Work out the finished part from the listing and answer in its coordinate system (mm). Face numbers are marked on the shaded views. A direction names the side the tool comes from. Round coordinates to 2 decimals unless told otherwise and drop trailing zeros. Loops run counter-clockwise (first coordinate to the right, second up) from the corner with the lowest first, then second, coordinate; pieces in that order, holes last. Notation, with made-up numbers: (-3, 65.5) - (6, 65.5) arc R7 ccw to (6, 75.5) - close; hole circle Ø11 at (-4.5, -13). An arc over 180 degrees is marked (long way). Answer as CSV lines item,"result". Start each with the question number.
```python
from build123d import *

# Parameters (mm, degrees)
F1_DEPTH = 1500
F2_R     = 120
F3_DEPTH = 715
F4_R     = 50


with BuildPart() as f1:
    # F0 (on Right) → F1 (new body)
    with BuildSketch(Plane.YZ):
        Polygon((250, 724.072175), (0, 724.072175), (-250, 724.072175), (-250, 524.072175), (-500, 524.072175), (-500, 124.072175), (-250, 124.072175), (-250, 324.072175), (0, 324.072175), (250, 324.072175), (250, 124.072175), (500, 124.072175), (500, 524.072175), (250, 524.072175), align=None)
    extrude(amount=F1_DEPTH)

    # F2 (on face) → F3 (cut)
    with BuildSketch(Plane.XY.offset(724.072175)):
        with Locations((300, 0)):
            Circle(F2_R)
        with Locations((1200, 0)):
            Circle(F2_R)
    extrude(amount=-F3_DEPTH, mode=Mode.SUBTRACT)

    # F4
    f4_edges = [f1.edges().sort_by_distance(p)[0] for p in [
        (750, -500, 524.072175),
        (750, 500, 524.072175),
    ]]
    fillet(f4_edges, radius=F4_R)


solid = f1.part
```
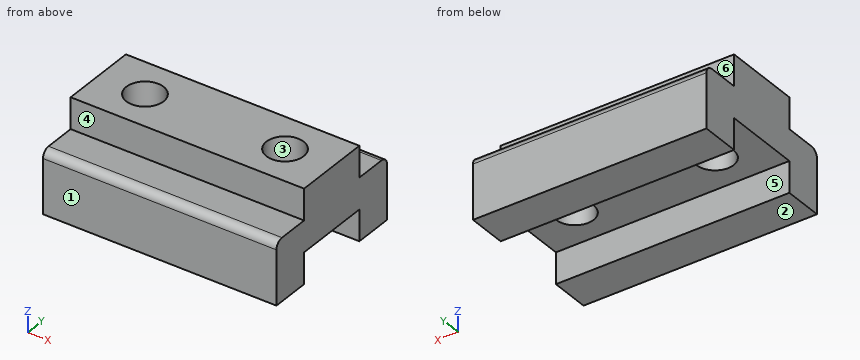
Item 1: Section D-D, the plane z = 306 is taken. Give the vertices of the cut face in (x, y).
Item 2: Section B-B, the plane y = 0 is taken. Give the vertices of the cut face in (x, z).
Item 3: Which of the six approach directions +Z, -Z, +X, -X, +Y, -Y give full straight-line access (tool end or side, diameter ignored) to the marked faces 4, 5 and 6?
Item 4: Flat-ended cylindrical pins translate along their axes: pin 1 Ø1.5 at (x, y) = (1002.5, 231.5) entering from -Z; pin 2 Ø1.5 at (x, z) = (282, 648) entering from +Y; pin 3 Ø8 at (x, y) = (1086, 36.5) entering from +Z. Find the tip coordinate at first contact, or state that the pin passes through.
Item 5: Determine the mould class of the marked faces 1, 2 and 3 for opening direction Y: pulls with the +Y half, pulls with the -Y half, needs draft (parallel to the pull), parting line crosses it, or undercut.
Item 6: Section C-C, the plane z = 542 is taken. Give the vertices of the cut face in (x, y), and give its area (3 significant figures).
Item 7: Find the intervals of material crossed by L1, parallel to Y at x = 300, z = 635; L2, parallel to Y at x = 334, z = 149; L3, parallel to X at y = 41, z = 382.5, in increasing order.
Item 8: Section A-A, the plane x = 300 is taken. Give the vertices of the cut face in (y, z).
Answer:
1,outline,"(0, -500) - (1500, -500) - (1500, -250) - (0, -250) - close; (0, 250) - (1500, 250) - (1500, 500) - (0, 500) - close"
2,outline,"(0, 324.07) - (180, 324.07) - (180, 724.07) - (0, 724.07) - close; (420, 324.07) - (1080, 324.07) - (1080, 724.07) - (420, 724.07) - close; (1320, 324.07) - (1500, 324.07) - (1500, 724.07) - (1320, 724.07) - close"
3,face 4,"+Z, +X, -X, -Y"
3,face 5,"-Z, +X, -X"
3,face 6,"+Z, +X, -X, +Y"
4,pin 1,"stops at z = 324.07"
4,pin 2,"stops at y = 250"
4,pin 3,"stops at z = 724.07"
5,face 1,"pulls with the -Y half"
5,face 2,"needs draft"
5,face 3,"undercut"
6,outline,"(0, -250) - (1500, -250) - (1500, 250) - (0, 250) - close; hole circle Ø240 at (300, 0); hole circle Ø240 at (1200, 0)"
6,area,"660,000 mm²"
7,L1,"y = -250 to -120, 120 to 250"
7,L2,"y = -500 to -250, 250 to 500"
7,L3,"x = 0 to 187.22, 412.78 to 1087.22, 1312.78 to 1500"
8,outline,"(-500, 124.07) - (-250, 124.07) - (-250, 324.07) - (-120, 324.07) - (-120, 724.07) - (-250, 724.07) - (-250, 524.07) - (-450, 524.07) arc R50 ccw to (-500, 474.07) - close; (120, 324.07) - (250, 324.07) - (250, 124.07) - (500, 124.07) - (500, 474.07) arc R50 ccw to (450, 524.07) - (250, 524.07) - (250, 724.07) - (120, 724.07) - close"
